from build123d import *

# Parameters (mm, degrees)
SKETCH1_R           = 38.1
BOSS_EXTRUDE3_DEPTH = 2.54


with BuildPart() as part:
    # Sketch1 → Boss-Extrude3 (new body)
    with BuildSketch(Plane(origin=(0, 0, 0), x_dir=(1, 0, 0), z_dir=(0, 1, 0))):
        with Locations(Location((-25.836673929, 73.693240411, 0), (0, 0, 270))):  # turned: the seam where the file's is
            Circle(SKETCH1_R)
        with BuildLine():
            Line((6.124442357, 89.281718391), (2.243449665, 87.388831779))
            ThreePointArc((2.243449665, 87.388831779), (-0.561364991, 92.056827263), (-4.134157119, 96.166854453))
            Line((-4.134157119, 96.166854453), (-1.134622276, 99.272963711))
            ThreePointArc((-1.134622276, 99.272963711), (2.931970391, 94.594883983), (6.124442357, 89.281718391))
        make_face(mode=Mode.SUBTRACT)
        with BuildLine():
            Line((-4.935030358, 102.461884731), (-7.473087077, 98.968549349))
            ThreePointArc((-7.473087077, 98.968549349), (-9.26937735, 100.180732706), (-11.145376456, 101.265479032))
            Line((-11.145376456, 101.265479032), (-9.114871927, 105.07627624))
            ThreePointArc((-9.114871927, 105.07627624), (-6.979588392, 103.841605625), (-4.935030358, 102.461884731))
        make_face(mode=Mode.SUBTRACT)
        with BuildLine():
            Line((9.183089768, 67.518311213), (4.930689891, 68.268124045))
            ThreePointArc((4.930689891, 68.268124045), (5.405326071, 73.693240411), (4.930689891, 79.118356778))
            Line((4.930689891, 79.118356778), (9.183089768, 79.868169609))
            ThreePointArc((9.183089768, 79.868169609), (9.723326071, 73.693240411), (9.183089768, 67.518311213))
        make_face(mode=Mode.SUBTRACT)
        with BuildLine():
            Line((7.98289579, 84.681884731), (3.876233753, 83.347549349))
            ThreePointArc((3.876233753, 83.347549349), (3.135507895, 85.384059217), (2.25539063, 87.364322037))
            Line((2.25539063, 87.364322037), (6.138033699, 89.253821123))
            ThreePointArc((6.138033699, 89.253821123), (7.139793188, 86.999863442), (7.98289579, 84.681884731))
        make_face(mode=Mode.SUBTRACT)
        with BuildLine():
            Line((-1.134622276, 48.113517111), (-4.134157119, 51.219626369))
            ThreePointArc((-4.134157119, 51.219626369), (-0.561364991, 55.329653559), (2.243449665, 59.997649043))
            Line((2.243449665, 59.997649043), (6.124442357, 58.104762431))
            ThreePointArc((6.124442357, 58.104762431), (2.931970391, 52.79159684), (-1.134622276, 48.113517111))
        make_face(mode=Mode.SUBTRACT)
        with BuildLine():
            Line((7.98289579, 62.704596091), (3.876233753, 64.038931473))
            ThreePointArc((3.876233753, 64.038931473), (4.474004412, 66.1218903), (4.925943869, 68.241276524))
            Line((4.925943869, 68.241276524), (9.177687792, 67.487753059))
            ThreePointArc((9.177687792, 67.487753059), (8.663285158, 65.075443537), (7.98289579, 62.704596091))
        make_face(mode=Mode.SUBTRACT)
        with BuildLine():
            Line((-20.887678459, 38.479307887), (-21.488627909, 42.755285408))
            ThreePointArc((-21.488627909, 42.755285408), (-16.182364991, 43.980332729), (-11.169443364, 46.108191715))
            Line((-11.169443364, 46.108191715), (-9.142265156, 42.295624009))
            ThreePointArc((-9.142265156, 42.295624009), (-14.848029609, 39.873670692), (-20.887678459, 38.479307887))
        make_face(mode=Mode.SUBTRACT)
        with BuildLine():
            Line((-4.935030358, 44.924596091), (-7.473087077, 48.417931473))
            ThreePointArc((-7.473087077, 48.417931473), (-5.765147975, 49.751719785), (-4.153777308, 51.20069591))
            Line((-4.153777308, 51.20069591), (-1.156954198, 48.091970247))
            ThreePointArc((-1.156954198, 48.091970247), (-2.991034632, 46.44272913), (-4.935030358, 44.924596091))
        make_face(mode=Mode.SUBTRACT)
        with BuildLine():
            Line((-42.531082702, 42.295624009), (-40.503904494, 46.108191715))
            ThreePointArc((-40.503904494, 46.108191715), (-35.490982867, 43.980332729), (-30.184719949, 42.755285408))
            Line((-30.184719949, 42.755285408), (-30.785669399, 38.479307887))
            ThreePointArc((-30.785669399, 38.479307887), (-36.825318249, 39.873670692), (-42.531082702, 42.295624009))
        make_face(mode=Mode.SUBTRACT)
        with BuildLine():
            Line((-25.836673929, 38.133240411), (-25.836673929, 42.451240411))
            ThreePointArc((-25.836673929, 42.451240411), (-23.670941071, 42.526396407), (-21.51562802, 42.751502802))
            Line((-21.51562802, 42.751502802), (-20.918410293, 38.475002482))
            ThreePointArc((-20.918410293, 38.475002482), (-23.371612139, 38.218783821), (-25.836673929, 38.133240411))
        make_face(mode=Mode.SUBTRACT)
        with BuildLine():
            Line((-57.797790215, 58.104762431), (-53.916797524, 59.997649043))
            ThreePointArc((-53.916797524, 59.997649043), (-51.111982867, 55.329653559), (-47.539190739, 51.219626369))
            Line((-47.539190739, 51.219626369), (-50.538725583, 48.113517111))
            ThreePointArc((-50.538725583, 48.113517111), (-54.605318249, 52.79159684), (-57.797790215, 58.104762431))
        make_face(mode=Mode.SUBTRACT)
        with BuildLine():
            Line((-46.738317501, 44.924596091), (-44.200260781, 48.417931473))
            ThreePointArc((-44.200260781, 48.417931473), (-42.403970508, 47.205748116), (-40.527971402, 46.12100179))
            Line((-40.527971402, 46.12100179), (-42.558475931, 42.310204583))
            ThreePointArc((-42.558475931, 42.310204583), (-44.693759466, 43.544875197), (-46.738317501, 44.924596091))
        make_face(mode=Mode.SUBTRACT)
        with BuildLine():
            Line((-60.856437626, 79.868169609), (-56.604037749, 79.118356778))
            ThreePointArc((-56.604037749, 79.118356778), (-57.078673929, 73.693240411), (-56.604037749, 68.268124045))
            Line((-56.604037749, 68.268124045), (-60.856437626, 67.518311213))
            ThreePointArc((-60.856437626, 67.518311213), (-61.396673929, 73.693240411), (-60.856437626, 79.868169609))
        make_face(mode=Mode.SUBTRACT)
        with BuildLine():
            Line((-59.656243648, 62.704596091), (-55.549581611, 64.038931473))
            ThreePointArc((-55.549581611, 64.038931473), (-54.808855753, 62.002421606), (-53.928738488, 60.022158786))
            Line((-53.928738488, 60.022158786), (-57.811381557, 58.132659699))
            ThreePointArc((-57.811381557, 58.132659699), (-58.813141046, 60.38661738), (-59.656243648, 62.704596091))
        make_face(mode=Mode.SUBTRACT)
        with BuildLine():
            Line((-50.538725583, 99.272963711), (-47.539190739, 96.166854453))
            ThreePointArc((-47.539190739, 96.166854453), (-51.111982867, 92.056827263), (-53.916797524, 87.388831779))
            Line((-53.916797524, 87.388831779), (-57.797790215, 89.281718391))
            ThreePointArc((-57.797790215, 89.281718391), (-54.605318249, 94.594883983), (-50.538725583, 99.272963711))
        make_face(mode=Mode.SUBTRACT)
        with BuildLine():
            Line((-59.656243648, 84.681884731), (-55.549581611, 83.347549349))
            ThreePointArc((-55.549581611, 83.347549349), (-56.14735227, 81.264590522), (-56.599291727, 79.145204299))
            Line((-56.599291727, 79.145204299), (-60.85103565, 79.898727763))
            ThreePointArc((-60.85103565, 79.898727763), (-60.336633016, 82.311037286), (-59.656243648, 84.681884731))
        make_face(mode=Mode.SUBTRACT)
        with BuildLine():
            Line((-30.785669399, 108.907172936), (-30.184719949, 104.631195415))
            ThreePointArc((-30.184719949, 104.631195415), (-35.490982867, 103.406148093), (-40.503904494, 101.278289107))
            Line((-40.503904494, 101.278289107), (-42.531082702, 105.090856813))
            ThreePointArc((-42.531082702, 105.090856813), (-36.825318249, 107.512810131), (-30.785669399, 108.907172936))
        make_face(mode=Mode.SUBTRACT)
        with BuildLine():
            Line((-46.738317501, 102.461884731), (-44.200260781, 98.968549349))
            ThreePointArc((-44.200260781, 98.968549349), (-45.908199883, 97.634761037), (-47.51957055, 96.185784912))
            Line((-47.51957055, 96.185784912), (-50.51639366, 99.294510575))
            ThreePointArc((-50.51639366, 99.294510575), (-48.682313226, 100.943751693), (-46.738317501, 102.461884731))
        make_face(mode=Mode.SUBTRACT)
        with BuildLine():
            Line((-25.836673929, 109.253240411), (-25.836673929, 104.935240411))
            ThreePointArc((-25.836673929, 104.935240411), (-28.002406787, 104.860084415), (-30.157719838, 104.63497802))
            Line((-30.157719838, 104.63497802), (-30.754937565, 108.91147834))
            ThreePointArc((-30.754937565, 108.91147834), (-28.301735719, 109.167697001), (-25.836673929, 109.253240411))
        make_face(mode=Mode.SUBTRACT)
        with BuildLine():
            Line((-20.887678459, 108.907172936), (-21.488627909, 104.631195415))
            ThreePointArc((-21.488627909, 104.631195415), (-16.182364991, 103.406148093), (-11.169443364, 101.278289107))
            Line((-11.169443364, 101.278289107), (-9.142265156, 105.090856813))
            ThreePointArc((-9.142265156, 105.090856813), (-14.848029609, 107.512810131), (-20.887678459, 108.907172936))
        make_face(mode=Mode.SUBTRACT)
    extrude(amount=BOSS_EXTRUDE3_DEPTH)


solid = part.part
Input: part model. Units: mm. Frame: model coordinates. Coordinates: 2 decimals unless noted, no trailing zeros. Order: outer loops, then holes, each group sorted by start corner. A loop starts at its lowest first (then second) coordinate and runs counter-clockwise, first axis right, second up.
1. Ray query, line 1 along X through (y, z) = (0.8, -78.5); line 2 along Z through (x, y) = (-32, 1.25); line 3 along X through (y, z) = (0.6, -55.5). Return the intervals inside material, ascending.
Checked values:
line 1: x = -63.63 to -61.07, -56.71 to 5.03, 9.4 to 11.96
line 2: z = -111.29 to -108.72, -104.32 to -43.07, -38.67 to -36.1
line 3: x = -59.31 to -56.39, -51.23 to -0.44, 4.72 to 7.64
2. Draft query along Z for faces 1 (the cylindrical face through (-5.79, 1.25, -49.73)), 2 (the cylindrical face through (-36.908, 1.252, -107.486)), 3 (the cylindrical face through (-49.02, 1.25, -103.93)). Return one class per face: +Z half, -Z half, draft (parallel to the pull), parting line (faces both ways), or undercut.
Checked values:
face 1: undercut
face 2: undercut
face 3: parting line
3. Cut plane C-C, the plane z = -40. Count the separate pieces of the cut face and the enclosed holes in it, plus the area to 3 significant figures.
Checked values:
separate pieces: 4
enclosed holes: 0
area: 44.7 mm2
4. Contact query for flat-ended pins moving along their axis: P1, Ø3, axis at x = -33.5, z = -63, coming from the -Y side; P2, Ø0.8, axis at y = 2, z = -39.5, coming from the +X side. Output: stop coordinate, or through.
Checked values:
P1: stops at y = 0
P2: stops at x = -8.24
5. Cut plane B-B, the plane z = -77.5. Return loops of the section in (x, y).
Checked values:
outline: (-63.75, 0) - (-61.19, 0) - (-61.19, 2.54) - (-63.75, 2.54) - close; (-56.85, 0) - (5.17, 0) - (5.17, 2.54) - (-56.85, 2.54) - close; (9.52, 0) - (12.07, 0) - (12.07, 2.54) - (9.52, 2.54) - close
6. Cut plane A-A, the plane x = -6. Return loops of the section in (y, z), plus the area to 3 significant figures.
Checked values:
outline: (0, -106.22) - (2.54, -106.22) - (2.54, -103.21) - (0, -103.21) - close; (0, -101) - (2.54, -101) - (2.54, -49.56) - (0, -49.56) - close; (0, -46.39) - (2.54, -46.39) - (2.54, -41.16) - (0, -41.16) - close
area: 152 mm2
